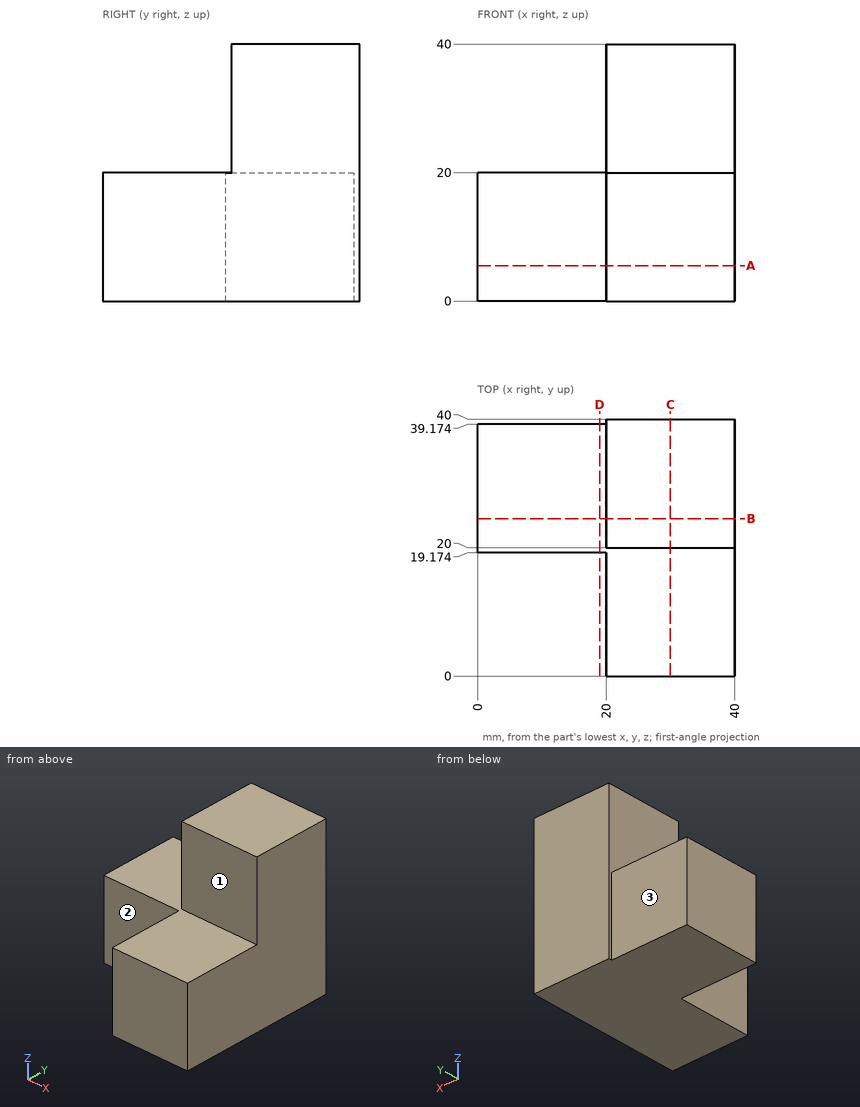
Part print with two shaded views. Sizes in mm from the minimum x, y, z corner. A direction names the side the tool comes from. Coordinates: 2 decimals unless noted, no trailing zeros. Order: outer loops, then holes, each group sorted by start corner. A loop starts at its lowest first (then second) coordinate and runs counter-clockwise, first axis right, second up.
(1) Saw through at A-A, the plane z = 5.5. Write the cut outline in (x, y).
Solution:
outline: (0, 19.17) - (20, 19.17) - (20, 0) - (40, 0) - (40, 40) - (20, 40) - (20, 39.17) - (0, 39.17) - close
(2) Saw through at B-B, the plane y = 24.5. Write the cut outline in (x, z).
Solution:
outline: (0, 0) - (40, 0) - (40, 40) - (20, 40) - (20, 20) - (0, 20) - close
(3) Which spindle directions (+Z, -Z, +X, -X, +Y, -Y) get a long thin tool onto all of the face, cutting with end or side? Do the marked faces 1, 2 and 3. Say none if no direction does.
Solution:
face 1: +Z, +X, -X, -Y
face 2: +Z, -Z, -X, -Y
face 3: +Z, -Z, -X, +Y
(4) Drill centre lines: L1, parallel to Z at x = 31, y = 7; L2, parallel to X at y = 21.5, z = 34.5. Where is each one in solid material? Low to high.
Solution:
L1: z = 0 to 20
L2: x = 20 to 40
(5) Saw through at D-D, the plane x = 19. Write the cut outline in (y, z).
Solution:
outline: (19.17, 0) - (39.17, 0) - (39.17, 20) - (19.17, 20) - close
(6) Pin check, flat tips, straight feed: pin 1 Ø10 at (x, z) = (25.5, 34.5) entering from -Y; pin 2 Ø10 at (x, z) = (10, 11) entering from -Y; pin 3 Ø15.5 at (y, z) = (9.5, 11.5) entering from -X. Stop position of each tip, or through.
Solution:
pin 1: stops at y = 20
pin 2: stops at y = 19.17
pin 3: stops at x = 20
